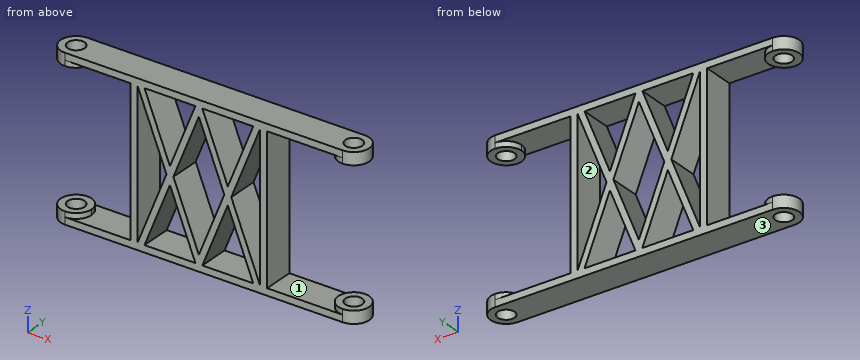
```python
from build123d import *

# Parameters (mm, degrees)
SKETCH1_R           = 11
BOSS_EXTRUDE1_DEPTH = 103.5
CUT_EXTRUDE1_REACH  = 230.719
SKETCH5_W           = 20
SKETCH5_H           = 175
FILLET1_R           = 20


with BuildPart() as part:
    # Sketch1 → Boss-Extrude1 (new, symmetric)
    with BuildSketch(Plane.XY):
        with BuildLine():
            Line((-180, -20), (180, -20))
            ThreePointArc((180, -20), (200, 0), (180, 20))
            Line((180, 20), (-180, 20))
            ThreePointArc((-180, 20), (-200, 0), (-180, -20))
        make_face()
        with Locations((-180, 0)):
            Circle(SKETCH1_R, mode=Mode.SUBTRACT)
        with Locations((180, 0)):
            Circle(SKETCH1_R, mode=Mode.SUBTRACT)
    extrude(amount=BOSS_EXTRUDE1_DEPTH, both=True)

    # Cut-Extrude1: up to this face of the body (flat: up to its plane)
    cut_extrude1_end = Plane(part.part.faces().sort_by_distance((0, -20, 0))[0])
    # Sketch5 → Cut-Extrude1 (cut, up to the picked face)
    with BuildSketch(Plane(origin=(0, 20, 0), x_dir=(1, 0, 0), z_dir=(0, 1, 0)), mode=Mode.PRIVATE) as cut_extrude1_sk1:
        Polygon((-95, -94.5), (-95, 94.5), (-160, 94.5), (-160, 87.5), (-180, 87.5), (-180, -87.5), (-160, -87.5), (-160, -94.5), align=None)
    cut_extrude1_tool1 = split(extrude(cut_extrude1_sk1.sketch, amount=-CUT_EXTRUDE1_REACH, mode=Mode.PRIVATE), bisect_by=cut_extrude1_end, keep=Keep.BOTH, mode=Mode.PRIVATE)
    # Sketch5 → Cut-Extrude1 (cut, up to the picked face)
    with BuildSketch(Plane(origin=(0, 20, 0), x_dir=(1, 0, 0), z_dir=(0, 1, 0)), mode=Mode.PRIVATE) as cut_extrude1_sk2:
        with Locations((-190, 0)):
            Rectangle(SKETCH5_W, SKETCH5_H)
    cut_extrude1_tool2 = split(extrude(cut_extrude1_sk2.sketch, amount=-CUT_EXTRUDE1_REACH, mode=Mode.PRIVATE), bisect_by=cut_extrude1_end, keep=Keep.BOTH, mode=Mode.PRIVATE)
    # Sketch5 → Cut-Extrude1 (cut, up to the picked face)
    with BuildSketch(Plane(origin=(0, 20, 0), x_dir=(1, 0, 0), z_dir=(0, 1, 0)), mode=Mode.PRIVATE) as cut_extrude1_sk3:
        Polygon((-48.5, 0), (-86, 94.5), (-86, -94.5), align=None)
    cut_extrude1_tool3 = split(extrude(cut_extrude1_sk3.sketch, amount=-CUT_EXTRUDE1_REACH, mode=Mode.PRIVATE), bisect_by=cut_extrude1_end, keep=Keep.BOTH, mode=Mode.PRIVATE)
    # Sketch5 → Cut-Extrude1 (cut, up to the picked face)
    with BuildSketch(Plane(origin=(0, 20, 0), x_dir=(1, 0, 0), z_dir=(0, 1, 0)), mode=Mode.PRIVATE) as cut_extrude1_sk4:
        Polygon((-11, 94.5), (-77, 94.5), (-44, 11.34), align=None)
    cut_extrude1_tool4 = split(extrude(cut_extrude1_sk4.sketch, amount=-CUT_EXTRUDE1_REACH, mode=Mode.PRIVATE), bisect_by=cut_extrude1_end, keep=Keep.BOTH, mode=Mode.PRIVATE)
    # Sketch5 → Cut-Extrude1 (cut, up to the picked face)
    with BuildSketch(Plane(origin=(0, 20, 0), x_dir=(1, 0, 0), z_dir=(0, 1, 0)), mode=Mode.PRIVATE) as cut_extrude1_sk5:
        Polygon((26.5, 0), (-6.5, 83.16), (-39.5, 0), (-6.5, -83.16), align=None)
    cut_extrude1_tool5 = split(extrude(cut_extrude1_sk5.sketch, amount=-CUT_EXTRUDE1_REACH, mode=Mode.PRIVATE), bisect_by=cut_extrude1_end, keep=Keep.BOTH, mode=Mode.PRIVATE)
    # Sketch5 → Cut-Extrude1 (cut, up to the picked face)
    with BuildSketch(Plane(origin=(0, 20, 0), x_dir=(1, 0, 0), z_dir=(0, 1, 0)), mode=Mode.PRIVATE) as cut_extrude1_sk6:
        Polygon((-44, -11.34), (-77, -94.5), (-11, -94.5), align=None)
    cut_extrude1_tool6 = split(extrude(cut_extrude1_sk6.sketch, amount=-CUT_EXTRUDE1_REACH, mode=Mode.PRIVATE), bisect_by=cut_extrude1_end, keep=Keep.BOTH, mode=Mode.PRIVATE)
    # Sketch5 → Cut-Extrude1 (cut, up to the picked face)
    with BuildSketch(Plane(origin=(0, 20, 0), x_dir=(1, 0, 0), z_dir=(0, 1, 0)), mode=Mode.PRIVATE) as cut_extrude1_sk7:
        Polygon((64, 94.5), (-2, 94.5), (31, 11.34), align=None)
    cut_extrude1_tool7 = split(extrude(cut_extrude1_sk7.sketch, amount=-CUT_EXTRUDE1_REACH, mode=Mode.PRIVATE), bisect_by=cut_extrude1_end, keep=Keep.BOTH, mode=Mode.PRIVATE)
    # Sketch5 → Cut-Extrude1 (cut, up to the picked face)
    with BuildSketch(Plane(origin=(0, 20, 0), x_dir=(1, 0, 0), z_dir=(0, 1, 0)), mode=Mode.PRIVATE) as cut_extrude1_sk8:
        Polygon((73, -94.5), (73, 94.5), (35.5, 0), align=None)
    cut_extrude1_tool8 = split(extrude(cut_extrude1_sk8.sketch, amount=-CUT_EXTRUDE1_REACH, mode=Mode.PRIVATE), bisect_by=cut_extrude1_end, keep=Keep.BOTH, mode=Mode.PRIVATE)
    # Sketch5 → Cut-Extrude1 (cut, up to the picked face)
    with BuildSketch(Plane(origin=(0, 20, 0), x_dir=(1, 0, 0), z_dir=(0, 1, 0)), mode=Mode.PRIVATE) as cut_extrude1_sk9:
        Polygon((31, -11.34), (-2, -94.5), (64, -94.5), align=None)
    cut_extrude1_tool9 = split(extrude(cut_extrude1_sk9.sketch, amount=-CUT_EXTRUDE1_REACH, mode=Mode.PRIVATE), bisect_by=cut_extrude1_end, keep=Keep.BOTH, mode=Mode.PRIVATE)
    # Sketch5 → Cut-Extrude1 (cut, up to the picked face)
    with BuildSketch(Plane(origin=(0, 20, 0), x_dir=(1, 0, 0), z_dir=(0, 1, 0)), mode=Mode.PRIVATE) as cut_extrude1_sk10:
        Polygon((160, 87.5), (160, 94.5), (82, 94.5), (82, -94.5), (160, -94.5), (160, -87.5), (180, -87.5), (180, 87.5), align=None)
    cut_extrude1_tool10 = split(extrude(cut_extrude1_sk10.sketch, amount=-CUT_EXTRUDE1_REACH, mode=Mode.PRIVATE), bisect_by=cut_extrude1_end, keep=Keep.BOTH, mode=Mode.PRIVATE)
    # Sketch5 → Cut-Extrude1 (cut, up to the picked face)
    with BuildSketch(Plane(origin=(0, 20, 0), x_dir=(1, 0, 0), z_dir=(0, 1, 0)), mode=Mode.PRIVATE) as cut_extrude1_sk11:
        with Locations((190, 0)):
            Rectangle(SKETCH5_W, SKETCH5_H)
    cut_extrude1_tool11 = split(extrude(cut_extrude1_sk11.sketch, amount=-CUT_EXTRUDE1_REACH, mode=Mode.PRIVATE), bisect_by=cut_extrude1_end, keep=Keep.BOTH, mode=Mode.PRIVATE)
    add(cut_extrude1_tool1.solids().sort_by(Axis((-136.923503, 20, 0), (0, -1, 0)))[0], mode=Mode.SUBTRACT)
    add(cut_extrude1_tool2.solids().sort_by(Axis((-190, 20, 0), (0, -1, 0)))[0], mode=Mode.SUBTRACT)
    add(cut_extrude1_tool3.solids().sort_by(Axis((-73.5, 20, 0), (0, -1, 0)))[0], mode=Mode.SUBTRACT)
    add(cut_extrude1_tool4.solids().sort_by(Axis((-44, 20, -66.78), (0, -1, 0)))[0], mode=Mode.SUBTRACT)
    add(cut_extrude1_tool5.solids().sort_by(Axis((-6.5, 20, 0), (0, -1, 0)))[0], mode=Mode.SUBTRACT)
    add(cut_extrude1_tool6.solids().sort_by(Axis((-44, 20, 66.78), (0, -1, 0)))[0], mode=Mode.SUBTRACT)
    add(cut_extrude1_tool7.solids().sort_by(Axis((31, 20, -66.78), (0, -1, 0)))[0], mode=Mode.SUBTRACT)
    add(cut_extrude1_tool8.solids().sort_by(Axis((60.5, 20, 0), (0, -1, 0)))[0], mode=Mode.SUBTRACT)
    add(cut_extrude1_tool9.solids().sort_by(Axis((31, 20, 66.78), (0, -1, 0)))[0], mode=Mode.SUBTRACT)
    add(cut_extrude1_tool10.solids().sort_by(Axis((130.401381, 20, 0), (0, -1, 0)))[0], mode=Mode.SUBTRACT)
    add(cut_extrude1_tool11.solids().sort_by(Axis((190, 20, 0), (0, -1, 0)))[0], mode=Mode.SUBTRACT)

    # Fillet1
    fillet1_edges = [part.edges().sort_by_distance(p)[0] for p in [
        (160, -20, 91),
        (160, 20, 91),
        (160, -20, -91),
        (160, 20, -91),
        (-160, -20, 91),
        (-160, 20, 91),
        (-160, -20, -91),
        (-160, 20, -91),
    ]]
    fillet(fillet1_edges, radius=FILLET1_R - 0.0001)  # a hair under: the kernel refuses the full size


solid = part.part
```
Verification items for the finished model (mm, model axes). Face numbers are marked on the shaded views. Coordinates: 2 decimals unless noted, no trailing zeros. Write each loop counter-clockwise with the first axis right and the second up, starting at its lowest first coordinate (ties: lowest second). Pieces come first, ordered by that corner, then holes. Notation, with made-up numbers: M -25,-6 L 8,-6 A22 ccw 8,13 Z; hole C 76.5,38 d8. An arc over 180 degrees is marked long. Answer as a JSON object with one key per item and string values. Group by question number.
(1) Cross-section at D-D, the plane x = -173. Record the cut outline in (y, z), and give its area (3 significant figures).
(2) Cross-section at A-A, the plane x = 55. Record the cut outline in (y, z).
(3) Cross-section at B-B, the plane z = -49. Record the cut outline in (x, y).
(4) Release check for a two-part mould opening along X. For the marked faces 1, 2 and 3 record: +X half, -X half, draft (parallel to the pull), parting line (faces both ways), or undercut.
(5) Cross-section at C-C, the plane y = 6.5. State how many separate pieces and enclosed holes the cut face has, and give its area (3 significant figures).
(6) Gauge pin test, flat ends, axial feed: pin 1 (12 mm diameter, centred on x = -182, y = -3.5, fed in from +Z); pin 2 (5 mm diameter, centred on y = -5, z = -39, fed in from -X); pin 3 (12 mm diameter, centred on x = -175.5, y = 7, fed in from -Z). Record the tip position at first contact, or that the pin passes through.
(7) Material ranges on line 1 (X direction, y = 0, z = -99); line 2 (Y direction, x = -180, z = -98); line 3 (Z direction, x = -141, y = -10.5), recorded low to high.
Reply:
{
 "1": {"outline": "M -20,-103.5 L -8.49,-103.5 L -8.49,-87.5 L -18.74,-87.5 L -18.74,-94.5 L -20,-94.5 Z; M -20,94.5 L -18.74,94.5 L -18.74,87.5 L -8.49,87.5 L -8.49,103.5 L -20,103.5 Z; M 8.49,-103.5 L 20,-103.5 L 20,-94.5 L 18.74,-94.5 L 18.74,-87.5 L 8.49,-87.5 Z; M 8.49,87.5 L 18.74,87.5 L 18.74,94.5 L 20,94.5 L 20,103.5 L 8.49,103.5 Z", "area": "702 mm²"},
 "2": {"outline": "M -20,-103.5 L 20,-103.5 L 20,-94.5 L -20,-94.5 Z; M -20,-71.82 L 20,-71.82 L 20,-49.14 L -20,-49.14 Z; M -20,49.14 L 20,49.14 L 20,71.82 L -20,71.82 Z; M -20,94.5 L 20,94.5 L 20,103.5 L -20,103.5 Z"},
 "3": {"outline": "M -95,-20 L -86,-20 L -86,20 L -95,20 Z; M -67.94,-20 L -58.94,-20 L -58.94,20 L -67.94,20 Z; M -29.06,-20 L -20.06,-20 L -20.06,20 L -29.06,20 Z; M 7.06,-20 L 16.06,-20 L 16.06,20 L 7.06,20 Z; M 45.94,-20 L 54.94,-20 L 54.94,20 L 45.94,20 Z; M 73,-20 L 82,-20 L 82,20 L 73,20 Z"},
 "4": {"face 1": "undercut", "face 2": "undercut", "face 3": "draft"},
 "5": {"separate pieces": "5", "enclosed holes": "7", "area": "17,000 mm²"},
 "6": {"pin 1": "through", "pin 2": "x = -95", "pin 3": "z = -103.5"},
 "7": {"line 1": "-200 to -191, -169 to 169, 191 to 200", "line 2": "-20 to -11, 11 to 20", "line 3": "-103.5 to -94.5, 94.5 to 103.5"}
}
